Could you check a few things on this model? Use its own coordinates, in mm. A direction names the side the tool comes from. Give positions to 0.01 mm unless a question says otherwise; leave off trailing zeros. Loops run counter-clockwise (first coordinate to the right, second up) from the corner with the lowest first, then second, coordinate; pieces in that order, holes last. Notation, with made-up numbers: M 65.25,-21 L 106.25,-21 A25 cw 106.25,5 Z; hole C 39.25,4.25 d10. An arc over 180 degrees is marked long. Write each question's results on one line, items separated by ' | '. Start each with the question number.
from build123d import *

# Parameters (mm, degrees)
SKETCH1_R           = 57.5
BOSS_EXTRUDE1_DEPTH = 10
SKETCH3_R           = 4.5
CUT_EXTRUDE2_DEPTH  = 10
SKETCH8_R           = 55
SKETCH8_R_2         = 53
CUT_EXTRUDE6_DEPTH  = 1.27
CIRPATTERN2_COUNT   = 4
HOLE1_D             = 5.5
HOLE1_DEPTH         = 10
HOLE1_CBORE_D       = 11
HOLE1_CBORE_DEPTH   = 5
CIRPATTERN3_COUNT   = 4


with BuildPart() as part:
    # Sketch1 → Boss-Extrude1 (new body)
    with BuildSketch(Plane.XY):
        Circle(SKETCH1_R)
    extrude(amount=BOSS_EXTRUDE1_DEPTH)

    # Sketch3 → Cut-Extrude2 (cut)
    with BuildSketch(Plane.XY.offset(10)):
        with Locations((0, -15)):
            Circle(SKETCH3_R)
        with Locations((10.606601718, 10.606601718)):
            Circle(SKETCH3_R)
        with Locations((-10.606601718, 10.606601718)):
            Circle(SKETCH3_R)
    extrude(amount=-CUT_EXTRUDE2_DEPTH, mode=Mode.SUBTRACT)

    # Sketch8 → Cut-Extrude6 (cut)
    with BuildSketch(Plane(origin=(0, 0, 0), x_dir=(-1, 0, 0), z_dir=(0, 0, -1))):
        Circle(SKETCH8_R)
        Circle(SKETCH8_R_2, mode=Mode.SUBTRACT)
    extrude(amount=-CUT_EXTRUDE6_DEPTH, mode=Mode.SUBTRACT)

    # Sketch10 → M3 Tapped Hole1 (revolve, cut)
    with BuildSketch(Plane(origin=(0, 54, 10), x_dir=(0, -1, 0), z_dir=(1, 0, 0))):
        Polygon((0, 0), (0, 7.251075774), (1.25, 6.5), (1.25, 0), align=None)
    m3_tapped_hole1 = revolve(axis=Axis((0, 54, 16.35), (0, 0, -1)), mode=Mode.SUBTRACT)

    # CirPattern2: M3 Tapped Hole1 ×4 about axis
    cirpattern2_axis = Axis((0, 0, 0), (0, 0, 1))
    for i in range(1, CIRPATTERN2_COUNT):
        add(m3_tapped_hole1.rotate(cirpattern2_axis, i * 360 / CIRPATTERN2_COUNT), mode=Mode.SUBTRACT)

    # Hole1
    with Locations(Plane.XY.offset(10)):
        with Locations((28.284271247, 28.284271247)):
            hole1 = CounterBoreHole(HOLE1_D / 2, HOLE1_CBORE_D / 2, HOLE1_CBORE_DEPTH, depth=HOLE1_DEPTH)

    # CirPattern3: Hole1 ×4 about axis
    cirpattern3_axis = Axis((0, 0, 0), (0, 0, 1))
    for i in range(1, CIRPATTERN3_COUNT):
        add(hole1.rotate(cirpattern3_axis, i * 360 / CIRPATTERN3_COUNT), mode=Mode.SUBTRACT)


solid = part.part
1) I'm going to push flat-ended pins straight in: P1, Ø3, axis at y = -7, z = 4, coming from the +X side; P2, Ø2, axis at x = 44.5, z = 8, coming from the +Y side; P3, Ø3.5, axis at x = 28, y = -27, coming from the +Z side. Where does each tip first touch, or does it pass through?
2) Thinking about a two-plate mould opening in X: for faces 4 (the face through (0.38, -52.81, 6.8)), 5 (the face through (14.763, 8.883, 5.07)), 6 (the face through (47, -30, 0)), which applies, pulls with the +X half, pulls with the -X half, needs draft (parallel to the pull), parting line crosses it, or undercut?
3) Which directions (+Z, -Z, +X, -X, +Y, -Y) give clear straight access to the entire face, cutting with the end or side of a thin tool? Please do faces 1 (the face through (-32, 24.23, 7.54)), 2 (the face through (-0.59, -10.54, 5.07)), 3 (the face through (11.923, -53.692, 0.626)).
4) If we section it at D-D on x = -12.5: Write out the boundary of the cut face in (y, z), plus the area to 3 significant figures.
5) If we section it at B-B on z = 7.75: State how many separate pieces and enclosed holes the cut face has, plus the area to 3 significant figures.
6) If we section it at A-A on x = 9.5: Write out the boundary of the cut face in (y, z).
7) If we section it at C-C on y = -36.5: Write out the boundary of the cut face in (x, z), plus the area to 3 significant figures.
8) Please list where these lines run through material, in increasing order: line 1 (X direction, y = 13.5, z = 7.25); line 2 (X direction, y = -17, z = 0.5); line 3 (X direction, y = -16, z = 0.75). Write a range as from..to.
Calculated:
1) P1: stops at x = 57.24 | P2: stops at y = 37.6 | P3: stops at z = 5
2) face 4: undercut | face 5: undercut | face 6: needs draft
3) face 1: +Z | face 2: +Z, -Z | face 3: -Z
4) outline: M -56.12,0 L -53.56,0 L -53.56,1.27 L -51.5,1.27 L -51.5,0 L 6.52,0 L 6.52,10 L -56.12,10 Z; M 14.69,0 L 51.5,0 L 51.5,1.27 L 53.56,1.27 L 53.56,0 L 56.12,0 L 56.12,10 L 14.69,10 Z | area: 1,040 mm2
5) separate pieces: 1 | enclosed holes: 11 | area: 9,800 mm2
6) outline: M -56.71,0 L -54.17,0 L -54.17,1.27 L -52.14,1.27 L -52.14,0 L 6.24,0 L 6.24,10 L -56.71,10 Z; M 14.97,0 L 52.14,0 L 52.14,1.27 L 54.17,1.27 L 54.17,0 L 56.71,0 L 56.71,10 L 14.97,10 Z
7) outline: M -44.43,0 L -41.14,0 L -41.14,1.27 L -38.43,1.27 L -38.43,0 L 38.43,0 L 38.43,1.27 L 41.14,1.27 L 41.14,0 L 44.43,0 L 44.43,10 L -44.43,10 Z | area: 882 mm2
8) line 1: x = -55.89..-14.05, -7.16..7.16, 14.05..55.89 | line 2: x = -54.93..-52.31, -50.2..-4.03, 4.03..50.2, 52.31..54.93 | line 3: x = -55.23..-52.62, -50.53..-4.39, 4.39..50.53, 52.62..55.23
